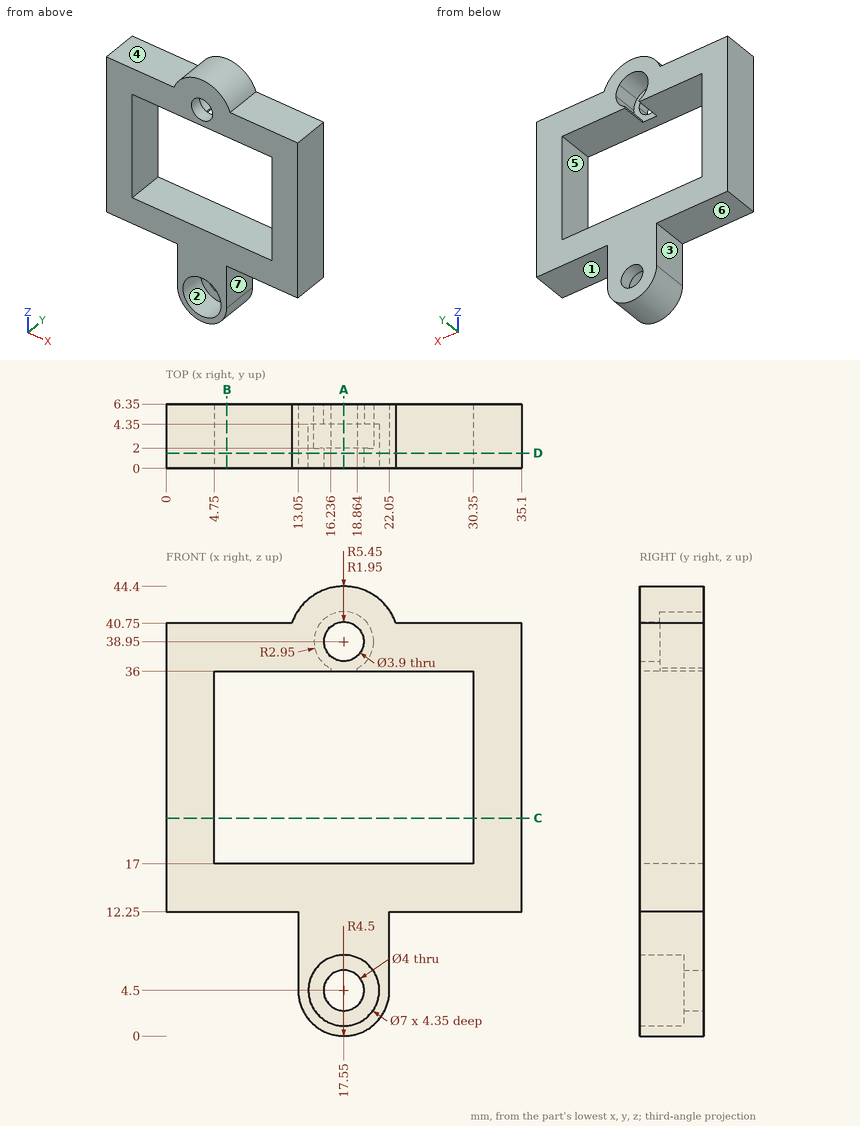
Design review of the part shown in the three views and the two pictorial views. Dimensions are in mm from the part's minimum x, y and z. A direction names the side the tool comes from. Give positions to 0.01 mm unless a question says otherwise; leave off trailing zeros. Write each loop counter-clockwise with the first axis right and the second up, starting at its lowest first coordinate (ties: lowest second). Pieces come first, ordered by that corner, then holes. Notation, with made-up numbers: M -10,54.25 L 27,54.25 A19 ccw 27,76.25 Z; hole C -18.5,51 d7. An arc over 180 degrees is marked long. One line per question, with ' | ' between items. Start each with the question number.
Item 1: For pin 1 (10 mm diameter, centred on x = 16, z = 26.5, fed in from +Y); pin 2 (1 mm diameter, centred on y = 5, z = 8, fed in from -X); pin 3 (1 mm diameter, centred on y = 4.5, z = 8.5, fed in from +X); pin 4 (1.9 mm diameter, centred on x = 7, y = 3.5, fed in from +Z), all flat-tipped, find the tip position at first contact; note any pin that passes through.
Item 2: We need section A-A on x = 17.55. Write out the cut boundary in (y, z).
Item 3: We need section B-B on x = 6. Write out the cut boundary in (y, z).
Item 4: Draft analysis for pull direction Z (two halves, no side actions). For the marked faces 1, 2, 3 and 4, state which applies: released by +Z, released by -Z, zero draft, split by the parting line, or undercut.
Item 5: We need section D-D on y = 1.5. Give the number of separate pieces and of enclosed holes in the cut face.
Item 6: We need section C-C on z = 21.5. Write out the cut boundary in (x, y).
Item 7: Wall thickness on line 1 (Z direction, x = 17.55, y = 1.35); line 2 (X direction, y = 1, z = 29.5); line 3 (X direction, y = 1.45, z = 38.95): over which ranges is each line inside the solid? List them lowest first. Write a range as from..to.
Item 8: For the marked faces 5, 6 and 7, list the 3-axis set-ups (+Z, -Z, +X, -X, +Y, -Y) from which the entire face can be reached by the end or side of a thin tool; tool diameter is ignored.
Results found:
1) pin 1: passes through | pin 2: stops at x = 13.05 | pin 3: stops at x = 22.05 | pin 4: stops at z = 40.75
2) outline: M 0,0 L 6.35,0 L 6.35,2.5 L 4.35,2.5 L 4.35,1 L 0,1 Z; M 0,8 L 4.35,8 L 4.35,6.5 L 6.35,6.5 L 6.35,17 L 0,17 Z; M 0,36 L 2,36 L 2,37 L 0,37 Z; M 0,40.9 L 2,40.9 L 2,41.9 L 6.35,41.9 L 6.35,44.4 L 0,44.4 Z
3) outline: M 0,12.25 L 6.35,12.25 L 6.35,17 L 0,17 Z; M 0,36 L 6.35,36 L 6.35,40.75 L 0,40.75 Z
4) face 1: released by -Z | face 2: undercut | face 3: zero draft | face 4: released by +Z
5) separate pieces: 1 | enclosed holes: 3
6) outline: M 0,0 L 4.75,0 L 4.75,6.35 L 0,6.35 Z; M 30.35,0 L 35.1,0 L 35.1,6.35 L 30.35,6.35 Z
7) line 1: z = 0..1, 8..17, 36..37, 40.9..44.4 | line 2: x = 0..4.75, 30.35..35.1 | line 3: x = 0..15.6, 19.5..35.1
8) face 5: +Y, -Y | face 6: -Z, -X, +Y, -Y | face 7: -Z, +X, +Y, -Y
